Autodesk Inventor part; units mm, degrees
ref_plane "YZ Plane" through (0, 0, 0) normal (1, 0, 0) x (0, 1, 0)
ref_plane "XZ Plane" through (0, 0, 0) normal (0, 1, 0) x (-1, 0, 0)
ref_plane "XY Plane" through (0, 0, 0) normal (0, 0, 1) x (1, 0, 0)
sketch "Sketch1" plane through (0, 0, 0) normal (1, 0, 0) x (0, 1, 0)
  line L0 (-4.2955, 0) -> (4.2955, 0)
  line L1 (0, 35) -> (0, 28.0784)
  line L2 (-2.5784, 25.25) -> (-5, 25.25)
  line L3 (-5, 25.25) -> (-5, 35)
  line L4 (-5, 35) -> (0, 35)
  line L5 (-2.5784, 25.25) -> (-0.25, 27.5784)
  line L6 (-0.25, 27.5784) -> (-0.25, 28.0784)
  line L7 (-0.25, 28.0784) -> (0, 28.0784)
  line L8 (0, 22.1716) -> (-2.8284, 25) construction
  line L9 (-2.8284, 25) -> (0, 27.8284) construction
  line L10 (0, 27.8284) -> (2.8284, 25) construction
  line L11 (2.8284, 25) -> (0, 22.1716) construction
  line L12 (0, 22.1716) -> (0, 27.8284) construction
  line L13 (-2.8284, 25) -> (2.8284, 25) construction
  point P0 (0, 0)
  point P1 (0, 0)
  point P2 (0, 25)
  point P3 (-1.4142, 26.4142)
  dimension "d1" = 5
  dimension "d2" = 0.5
  dimension "d3" = 0.25
  dimension "d4" = 135
  dimension "d7" = 4
  dimension "d8" = 50
  dimension "d9" = 0.25
  dimension "d10" = 70
revolve "Revolution1" add sketch "Sketch1" angle 360 about axis through (0, -4.2955, 0) along (0, 1, 0)
sketch "Sketch3" plane through (0, -5, 0) normal (0, -1, 0) x (1, 0, 0)
  circle A0 centre (0, 0) radius 35
  arc A1 (2.5275, 28.8896) -> (-2.5275, 28.8896) centre (0, 0) ccw construction
  arc A2 (2.2508, 25.7267) -> (-2.2508, 25.7267) centre (0, 0) ccw
  arc A3 (2.2508, 25.7267) -> (5.3051, 27.3516) centre (2.5275, 28.8896) ccw
  arc A4 (-5.3051, 27.3516) -> (-2.2508, 25.7267) centre (-2.5275, 28.8896) ccw
  line L0 (2.5275, 28.8896) -> (0, 0) construction
  line L1 (0, 0) -> (-2.5275, 28.8896) construction
  arc A5 (7.0816, 28.1221) -> (5.3051, 27.3516) centre (6.6939, 26.5826) ccw
  arc A6 (-5.3051, 27.3516) -> (-7.0816, 28.1221) centre (-6.6939, 26.5826) ccw
  arc A7 (-25.7267, 2.2508) -> (-27.3516, 5.3051) centre (-28.8896, 2.5275) ccw
  arc A8 (-28.1221, 7.0816) -> (-27.3516, 5.3051) centre (-26.5826, 6.6939) ccw
  arc A9 (-27.3516, -5.3051) -> (-28.1221, -7.0816) centre (-26.5826, -6.6939) ccw
  arc A10 (-27.3516, -5.3051) -> (-25.7267, -2.2508) centre (-28.8896, -2.5275) ccw
  arc A11 (-25.7267, 2.2508) -> (-25.7267, -2.2508) centre (0, 0) ccw
  arc A12 (-2.2508, -25.7267) -> (-5.3051, -27.3516) centre (-2.5275, -28.8896) ccw
  arc A13 (-7.0816, -28.1221) -> (-5.3051, -27.3516) centre (-6.6939, -26.5826) ccw
  arc A14 (5.3051, -27.3516) -> (7.0816, -28.1221) centre (6.6939, -26.5826) ccw
  arc A15 (5.3051, -27.3516) -> (2.2508, -25.7267) centre (2.5275, -28.8896) ccw
  arc A16 (-2.2508, -25.7267) -> (2.2508, -25.7267) centre (0, 0) ccw
  arc A17 (25.7267, -2.2508) -> (27.3516, -5.3051) centre (28.8896, -2.5275) ccw
  arc A18 (28.1221, -7.0816) -> (27.3516, -5.3051) centre (26.5826, -6.6939) ccw
  arc A19 (27.3516, 5.3051) -> (28.1221, 7.0816) centre (26.5826, 6.6939) ccw
  arc A20 (27.3516, 5.3051) -> (25.7267, 2.2508) centre (28.8896, 2.5275) ccw
  arc A21 (25.7267, -2.2508) -> (25.7267, 2.2508) centre (0, 0) ccw
  arc A22 (-7.0816, 28.1221) -> (-28.1221, 7.0816) centre (0, 0) ccw
  arc A23 (-28.1221, -7.0816) -> (-7.0816, -28.1221) centre (0, 0) ccw
  arc A24 (7.0816, -28.1221) -> (28.1221, -7.0816) centre (0, 0) ccw
  arc A25 (28.1221, 7.0816) -> (7.0816, 28.1221) centre (0, 0) ccw
  point P0 (0, 29)
  dimension "d13" = 70
  dimension "d16" = 10
  dimension "d17" = 3.175
  dimension "d18" = 1.5875
  dimension "d21" = 360
  dimension "d23" = 29
extrude "Extrusion1" add sketch "Sketch3" along normal blind 1.5
sketch "Sketch6" plane through (0, 0, 0) normal (0, 1, 0) x (1, 0, 0)
  circle A0 centre (0, 0) radius 35
  line L0 (0, -35) -> (0, 0)
  point P0 (0, -32)
  point P1 (32, 0)
  point P2 (0, 32)
  point P3 (-32, 0)
  dimension "d47" = 3
  dimension "d50" = 360
hole "Hole2" at (0, 0, 32) at (32, 0, 0) at (0, 0, -32) at (-32, 0, 0) direction (0, -1, 0) diameter 3.2 end through all counterbore diameter 5 counterbore depth 1.5
sketch "Sketch5" plane through (0, -6.5, 0) normal (0, -1, 0) x (1, 0, 0)
  circle A0 centre (32, 0) radius 2.5
  line L0 (32, 0) -> (0, 0)
  line L1 (0, 0) -> (29.6429, -18.1652)
  point P0 (27.2845, -16.72)
  dimension "d32" = 31.5
  dimension "d33" = 32
hole "Hole1" at (27.2845, -6.5, -16.72) direction (0, 1, 0) diameter 3.242 end through all
pattern_circular "Circular Pattern1" count 2 over 27 about axis through (0, -2.5, 0) along (0, 1, 0) of "Hole1"
pattern_circular "Circular Pattern2" count 4 over 360 about axis through (0, -2.5, 0) along (0, 1, 0) of "Hole1", "Circular Pattern1"
properties part number "CR_OUTSIDE,BOTTOM,REV-ENG" material "Steel, A2, HT 56-58 Rc"
Geometry check sheet. Reference: the model listing, model coordinates, mm. A direction names the side the tool comes from. Round coordinates to 2 decimals unless told otherwise and drop trailing zeros. Loops run counter-clockwise (first coordinate to the right, second up) from the corner with the lowest first, then second, coordinate; pieces in that order, holes last. Notation, with made-up numbers: (-19.75, 22.5) - (34.25, 22.5) arc R19 cw to (34.25, 56.5) - close; hole circle Ø11 at (-11, 24.5). An arc over 180 degrees is marked (long way). Write item = value, one per line. Start each with the question number.
1. Section check A-A on z = -32. Enter the section's corners in (x, y), then the cut area to 3 significant figures.
2. Depth check by flat-ended pin: pin 1 (1.5 mm diameter, centred on x = -6.5, y = -5, fed in from -Z); pin 2 (2.5 mm diameter, centred on x = -33, z = -0.5, fed in from +Y); pin 3 (1.5 mm diameter, centred on x = 2, y = -5.5, fed in from +Z). Enter the tip coordinate at first touch or a pass-through.
3. Set-up check for faces 3 (the face through (28.045, -5.74, 6.076)), 4 (the face through (-0.07, -4.04, 30.4)), 5 (the face through (-32, -1.5, 2)): record each of +Z, -Z, +X, -X, +Y, -Y from which the full face is reachable in a straight line by a thin tool's end or side.
4. Section check C-C on y = -3.5. Give the number of separate pieces and of enclosed holes in the cut face, then the cut area to 3 significant figures.
5. Mould release check, pull along Z, two halves, no side actions. Record for faces 1 (the face through (-28.033, -5.74, 6.049)), 2 (the face through (-28.4, 0, -0.2)): released by +Z, released by -Z, zero draft, split by the parting line, or undercut.
6. Thickness scan on line 1 (X direction, y = -2.75, z = 0); line 2 (X direction, y = -1, z = -17); line 3 (Z direction, x = -18, y = -0.75). Record the ranges inside material, lowest first.
7. Section check B-B on x = -32. Enter the section's corners in (y, z).
Working result:
q1.outline = (-14.18, -6.5) - (-1.6, -6.5) - (-1.6, -1.5) - (-2.5, -1.5) - (-2.5, 0) - (-14.18, 0) - close; (1.6, -6.5) - (14.18, -6.5) - (14.18, 0) - (2.5, 0) - (2.5, -1.5) - (1.6, -1.5) - close
q1.area = 161 mm^2
q2.pin_1 = -34.52
q2.pin_2 = -1.5
q2.pin_3 = 34.98
q3.face_3 = -Y
q3.face_4 = +Y, -Y
q3.face_5 = +Y
q4.separate_pieces = 1
q4.enclosed_holes = 13
q4.area = 1,750 mm^2
q5.face_1 = undercut
q5.face_2 = zero draft
q6.line_1 = -35 to -33.6, -30.4 to -25.25, 25.25 to 30.4, 33.6 to 35
q6.line_2 = -30.59 to -28.88, -25.69 to -20.75, 20.75 to 25.69, 28.88 to 30.59
q6.line_3 = -30.02 to -28.28, -26.29 to -20.23, 20.23 to 26.29, 28.28 to 30.02
q7.outline = (-6.5, -14.18) - (0, -14.18) - (0, -2.5) - (-1.5, -2.5) - (-1.5, -1.6) - (-6.5, -1.6) - close; (-6.5, 1.6) - (-1.5, 1.6) - (-1.5, 2.5) - (0, 2.5) - (0, 14.18) - (-6.5, 14.18) - close
